Could you check a few things on this model? Use its own coordinates, in mm. Face numbers are marked on the shaded views. A direction names the side the tool comes from. Give positions to 0.01 mm unless a question says otherwise; leave off trailing zeros. Write each loop counter-clockwise with the first axis right and the second up, starting at its lowest first coordinate (ties: lowest second). Pieces come first, ordered by that corner, then holes. Notation, with made-up numbers: (-8.75, -33.75) - (34.25, -33.75) arc R19 ccw to (34.25, -28.75) - close; hole circle Ø3 at (86, 44). An arc over 180 degrees is marked (long way). Answer in a Markdown table with one row per item.
Autodesk Inventor part; units mm, degrees
ref_plane "YZ Plane" through (0, 0, 0) normal (1, 0, 0) x (0, 1, 0)
ref_plane "XZ Plane" through (0, 0, 0) normal (0, 1, 0) x (-1, 0, 0)
ref_plane "XY Plane" through (0, 0, 0) normal (0, 0, 1) x (1, 0, 0)
sketch "Esquisse1" plane through (0, 0, 0) normal (0, 0, 1) x (1, 0, 0)
  line L0 (0, 0) -> (42, 0)
  line L1 (42, 0) -> (42, 10.5)
  line L2 (42, 10.5) -> (0, 10.5)
  line L3 (0, 10.5) -> (0, 0)
  dimension "d0" = 42
  dimension "d1" = 10.5
extrude "Extrusion1" add sketch "Esquisse1" along normal blind 3
sketch "Esquisse2" plane through (0, 0, 3) normal (0, 0, 1) x (1, 0, 0)
  line L0 (0, 10.5) -> (0, 0)
  circle A0 centre (3, 5.25) radius 2
  circle A1 centre (13, 5.25) radius 2
  dimension "d4" = 3
  dimension "d5" = 10
  dimension "d6" = 4
  dimension "d7" = 4
extrude "Extrusion2" cut sketch "Esquisse2" against normal through all
sketch "Esquisse3" plane through (0, 0, 3) normal (0, 0, 1) x (1, 0, 0)
  line L0 (0, 10.5) -> (0, 0)
  line L1 (0, 10.5) -> (5.5, 10.5)
  line L2 (42, 10.5) -> (0, 10.5)
  line L3 (5.5, 10.5) -> (10.5, 10.5)
  line L4 (10.5, 10.5) -> (10.5, 0)
  line L5 (10.5, 0) -> (5.5, 0)
  line L6 (5.5, 0) -> (5.5, 10.5)
  dimension "d10" = 5.5
  dimension "d11" = 5
  dimension "d12" = 10.5
extrude "Extrusion3" add sketch "Esquisse3" along normal blind 4
sketch "Esquisse4" plane through (0, 0, 3) normal (0, 0, 1) x (1, 0, 0)
  line L0 (42, 10.5) -> (0, 10.5)
  line L1 (42, 10.5) -> (37, 10.5)
  line L2 (37, 10.5) -> (37, 0)
  line L3 (37, 0) -> (42, 0)
  line L4 (42, 0) -> (42, 10.5)
  point P0 (0, 0)
  dimension "d15" = 5
  dimension "d16" = 10.5
extrude "Extrusion4" add sketch "Esquisse4" along normal blind 5
sketch "Esquisse5" plane through (42, 0, 0) normal (1, 0, 0) x (0, 0, -1)
  line L0 (-8, 10.5) -> (-8, 0)
  line L1 (-8, 0) -> (-5, 0)
  line L2 (-5, 0) -> (-5, 2.5)
  line L3 (-5, 2.5) -> (-8, 2.5)
  line L4 (-8, 2.5) -> (-8, 0)
  line L5 (-8, 2.5) -> (-8, 4)
  line L6 (-8, 4) -> (-5, 4)
  line L7 (-5, 4) -> (-5, 6.5)
  line L8 (-5, 6.5) -> (-8, 6.5)
  line L9 (-8, 6.5) -> (-8, 4)
  line L10 (-8, 6.5) -> (-8, 8)
  line L11 (-8, 8) -> (-5, 8)
  line L12 (-5, 8) -> (-5, 10.5)
  line L13 (-5, 10.5) -> (-8, 10.5)
  line L14 (-8, 10.5) -> (-8, 8)
  point P0 (0, 0)
  dimension "d21" = 3
  dimension "d22" = 2.5
  dimension "d23" = 1.5
  dimension "d24" = 3
  dimension "d25" = 2.5
  dimension "d26" = 1.5
  dimension "d27" = 3
  dimension "d28" = 2.5
extrude "Extrusion5" add sketch "Esquisse5" along normal blind 5
sketch "Esquisse6" plane through (42, 0, 0) normal (1, 0, 0) x (0, 0, -1)
  line L0 (-5, 2.5) -> (-8, 2.5)
  line L1 (-5, 6.5) -> (-5, 4)
  line L2 (-8, 2.5) -> (-5, 2.5)
  line L3 (-5, 2.5) -> (-5, 4)
  line L4 (-5, 4) -> (-8, 4)
  line L5 (-8, 4) -> (-8, 2.5)
  line L6 (-8, 6.5) -> (-5, 6.5)
  line L7 (-5, 6.5) -> (-5, 8.0213)
  line L8 (-5, 8.0213) -> (-8, 8.0213)
  line L9 (-8, 8.0213) -> (-8, 6.5)
  point P0 (0, 0)
extrude "Extrusion6" cut sketch "Esquisse6" against normal blind 5
properties part number "IF - TCRT5000"
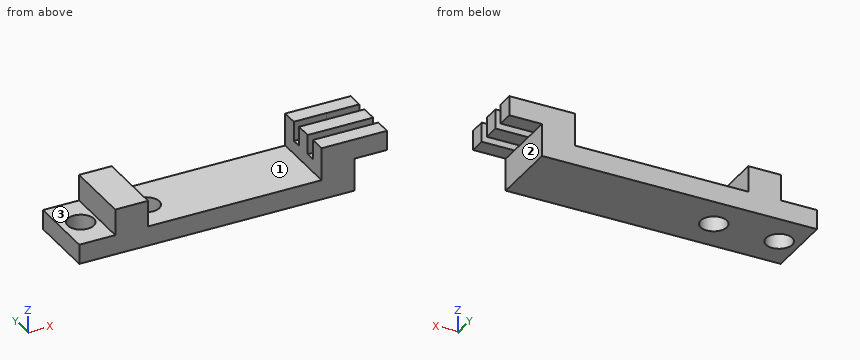
1) Imagine slicing it at D-D (x = 25). List the corners of the cut face in (y, z) for me.
Check values:
| item | result |
|---|---|
| outline | (0, 0) - (10.5, 0) - (10.5, 3) - (0, 3) - close |
2) If I drill on line 1 (Y direction, x = 3, z = 2); line 2 (X direction, y = 5.75, z = 2.25); line 3 (X direction, y = 5.5, z = 1.25), over which ranges is the centre line in solid material (lowest first)?
Check values:
| item | result |
|---|---|
| line 1 | y = 0 to 3.25, 7.25 to 10.5 |
| line 2 | x = 0 to 1.06, 4.94 to 11.06, 14.94 to 42 |
| line 3 | x = 0 to 1.02, 4.98 to 11.02, 14.98 to 42 |
3) On a 3-axis mill with a long thin cutter (end or side, diameter ignored), from which of +Z, -Z, +X, -X, +Y, -Y can I reach the whole of each face in a straight line? I mean the marked faces 1, 2 and 3. Say none if no direction works.
Check values:
| item | result |
|---|---|
| face 1 | +Z, +Y, -Y |
| face 2 | -Z, +X, +Y, -Y |
| face 3 | +Z, -X, +Y, -Y |
4) Imagine slicing it at B-B (y = 5.25). List the corners of the cut face in (x, z) for me.
Check values:
| item | result |
|---|---|
| outline | (0, 0) - (1, 0) - (1, 3) - (0, 3) - close; (5, 0) - (11, 0) - (11, 3) - (10.5, 3) - (10.5, 7) - (5.5, 7) - (5.5, 3) - (5, 3) - close; (15, 0) - (42, 0) - (42, 5) - (47, 5) - (47, 8) - (37, 8) - (37, 3) - (15, 3) - close |
5) Will these pins go through, and if not, where does the flat tip stop? P1, Ø0.9, axis at x = 43.5, z = 6, coming from the -Y side; P2, Ø1.5, axis at x = 10, y = 4, coming from the +Z side; P3, Ø2, axis at x = 43.5, y = 5, coming from the -Z side; P4, Ø2.5, axis at y = 7, z = 2, coming from the +X side.
Check values:
| item | result |
|---|---|
| P1 | stops at y = 0 |
| P2 | stops at z = 7 |
| P3 | stops at z = 5 |
| P4 | stops at x = 42 |
6) Imagine slicing it at A-A (x = 13). List the corners of the cut face in (y, z) for me, then the cut area to 3 significant figures.
Check values:
| item | result |
|---|---|
| outline | (0, 0) - (3.25, 0) - (3.25, 3) - (0, 3) - close; (7.25, 0) - (10.5, 0) - (10.5, 3) - (7.25, 3) - close |
| area | 19.5 mm2 |
7) Imagine slicing it at C-C (z = 1.5). List the corners of the cut face in (x, y) for me, then the cut area to 3 significant figures.
Check values:
| item | result |
|---|---|
| outline | (0, 0) - (42, 0) - (42, 10.5) - (0, 10.5) - close; hole circle Ø4 at (3, 5.25); hole circle Ø4 at (13, 5.25) |
| area | 416 mm2 |
